Read the model definition and answer for the solid it produces. Units are mm, in the model's axes. Face numbers are marked on the shaded views. A direction names the side the tool comes from. Give positions to 0.01 mm unless a question says otherwise; leave off trailing zeros. Loops run counter-clockwise (first coordinate to the right, second up) from the corner with the lowest first, then second, coordinate; pieces in that order, holes last. Notation, with made-up numbers: (-29.5, 54.5) - (-1.5, 54.5) arc R21 ccw to (-1.5, 90.5) - close; hole circle Ø5 at (50.5, 5). An arc over 180 degrees is marked (long way). Use a Markdown table: item, result. Add a question column.
Item 1: Each of these flat-tipped pins is pushed along its axis until it touches: P1, Ø1.9, axis at x = -4.5, y = 4, coming from the +Z side; P2, Ø8, axis at x = -2, y = 3, coming from the +Z side; P3, Ø12, axis at x = 6, z = 18.5, coming from the +Y side. Where does it stop, or does it pass through?
Item 2: A cutting plane is placed at C-C (y = -14). Determine the outline of the cut face in (x, z), plus the area to 3 significant figures.
Item 3: Which of the six approach directions +Z, -Z, +X, -X, +Y, -Y give full straight-line access (tool end or side, diameter ignored) to the marked faces 4 and 5?
Item 4: A cutting plane is placed at A-A (z = 7). Determine the outline of the cut face in (x, y).
Item 5: A cutting plane is placed at B-B (z = 22). Determine the outline of the cut face in (x, y).
Item 6: A cutting plane is placed at D-D (x = -5). Determine the outline of the cut face in (y, z), plus the area to 3 significant figures.
Item 7: Consider probe 1 along Y at (x, z) = (0, 5.25); probe 2 along X at (y, z) = (-27.65, 14); probe 3 along X at (y, z) = (-18, 13). Determine where each line is inside the solid, lowest interval first. Write a range as [from, to].
Item 8: For a pull along X with two mould halves and no side action, classify the marked faces 1, 2 and 3 as +X half, -X half, draft (parallel to the pull), parting line (faces both ways), or undercut.
from build123d import *

# Parameters (mm, degrees)
SKETCH1_R           = 6.5
BOSS_EXTRUDE1_DEPTH = 13
CUT_EXTRUDE1_DEPTH  = 2
SKETCH3_R           = 1
SKETCH3_W           = 13
SKETCH3_H           = 22
CUT_EXTRUDE2_DEPTH  = 9
BOSS_EXTRUDE2_DEPTH = 18
BOSS_EXTRUDE3_DEPTH = 1.5
BOSS_EXTRUDE4_DEPTH = 1.5
SKETCH7_R           = 2.5
SKETCH7_R_2         = 1.3
CUT_EXTRUDE3_DEPTH  = 5


with BuildPart() as part:
    # Sketch1 → Boss-Extrude1 (new body)
    with BuildSketch(Plane.XY):
        with BuildLine():
            Line((-16.5, 0), (-16.5, -29.5))
            Line((-16.5, -29.5), (16.5, -29.5))
            Line((16.5, -29.5), (16.5, 0))
            ThreePointArc((16.5, 0), (0, 16.5), (-16.5, 0))
        make_face()
        with Locations(Location((0, 0, 0), (0, 0, 180))):
            Circle(SKETCH1_R, mode=Mode.SUBTRACT)
    extrude(amount=BOSS_EXTRUDE1_DEPTH)

    # Sketch2 → Cut-Extrude1 (cut)
    with BuildSketch(Plane.XY.offset(13)):
        with BuildLine():
            Line((-13.5, -26.5), (13.5, -26.5))
            Line((13.5, -26.5), (13.5, 0))
            ThreePointArc((13.5, 0), (0, 13.5), (-13.5, 0))
            Line((-13.5, 0), (-13.5, -26.5))
        make_face()
    extrude(amount=-CUT_EXTRUDE1_DEPTH, mode=Mode.SUBTRACT)

    # Sketch3 → Cut-Extrude2 (cut)
    with BuildSketch(Plane.XY.offset(11)):
        with Locations((0, 9.3)):
            Circle(SKETCH3_R)
        with Locations(Location((0, -18.3, 0), (0, 0, 180))):
            Circle(SKETCH3_R)
        with Locations((0, -4.5)):
            Rectangle(SKETCH3_W, SKETCH3_H)
    extrude(amount=-CUT_EXTRUDE2_DEPTH, mode=Mode.SUBTRACT)

    # Sketch4 → Boss-Extrude2 (add)
    with BuildSketch(Plane.XY.offset(13)):
        Polygon((-16.5, -26.5), (-16.5, -29.5), (16.5, -29.5), (16.5, -26.5), (13.5, -26.5), (-13.5, -26.5), align=None)
    extrude(amount=BOSS_EXTRUDE2_DEPTH)

    # Sketch5 → Boss-Extrude3 (add, symmetric)
    with BuildSketch(Plane(origin=(-15, 0, 0), x_dir=(0, 0, -1), z_dir=(1, 0, 0))):
        Polygon((-13, 0), (-31, -26.5), (-13, -26.5), align=None)
    extrude(amount=BOSS_EXTRUDE3_DEPTH, both=True)

    # Sketch6 → Boss-Extrude4 (add, symmetric)
    with BuildSketch(Plane(origin=(15, 0, 0), x_dir=(0, 0, -1), z_dir=(1, 0, 0))):
        Polygon((-13, 0), (-31, -26.5), (-13, -26.5), align=None)
    extrude(amount=BOSS_EXTRUDE4_DEPTH, both=True)

    # Sketch7 → Cut-Extrude3 (cut)
    with BuildSketch(Plane.XZ.offset(29.5)):
        with Locations(Location((-5, 14, 0), (0, 0, 270))):
            Circle(SKETCH7_R)
        with Locations(Location((-0.5, 14, 0), (0, 0, 270))):
            Circle(SKETCH7_R_2)
        with Locations(Location((-9.5, 14, 0), (0, 0, 270))):
            Circle(SKETCH7_R_2)
    extrude(amount=-CUT_EXTRUDE3_DEPTH, mode=Mode.SUBTRACT)


solid = part.part
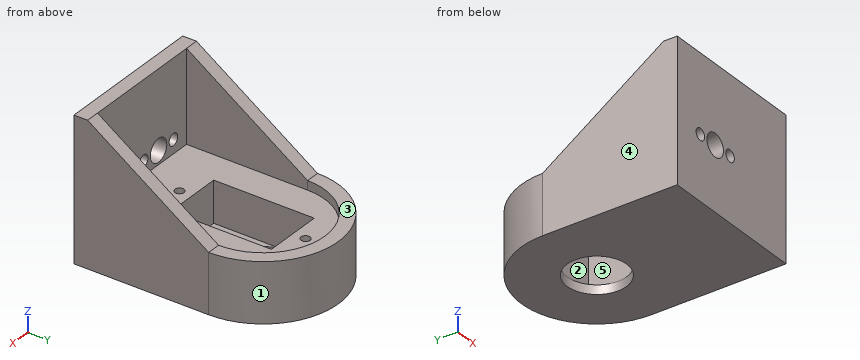
Geometry says:
| question | item | result |
|---|---|---|
| 1 | P1 | z = 2 |
| 1 | P2 | z = 11 |
| 1 | P3 | y = 16.1 |
| 2 | outline | (-16.5, 0) - (16.5, 0) - (16.5, 22.51) - (13.5, 22.51) - (13.5, 11) - (6.5, 11) - (6.5, 2) - (-6.5, 2) - (-6.5, 11) - (-13.5, 11) - (-13.5, 22.51) - (-16.5, 22.51) - close |
| 2 | area | 315 mm² |
| 3 | face 4 | +Z, -Z, -X, +Y, -Y |
| 3 | face 5 | +Z |
| 4 | outline | (-16.5, -29.5) - (16.5, -29.5) - (16.5, 0) arc R16.5 ccw to (-16.5, 0) - close; hole (-6.5, -15.5) - (6.5, -15.5) - (6.5, 6.5) - (-6.5, 6.5) - close; hole circle Ø2 at (0, -18.3); hole circle Ø2 at (0, 9.3) |
| 5 | outline | (-16.5, -29.5) - (16.5, -29.5) - (16.5, -13.25) - (13.5, -13.25) - (13.5, -26.5) - (-13.5, -26.5) - (-13.5, -13.25) - (-16.5, -13.25) - close |
| 6 | outline | (-29.5, 0) - (-4.15, 0) - (-4.15, 2) - (-15.5, 2) - (-15.5, 11) - (-26.5, 11) - (-26.5, 11.5) - (-29.5, 11.5) - close; (-29.5, 16.5) - (-26.5, 16.5) - (-26.5, 31) - (-29.5, 31) - close; (4.15, 0) - (15.72, 0) - (15.72, 13) - (12.54, 13) - (12.54, 11) - (6.5, 11) - (6.5, 2) - (4.15, 2) - close |
| 6 | area | 334 mm² |
| 7 | probe 1 | [-29.5, -19.3], [-17.3, -15.5], [6.5, 8.3], [10.3, 16.5] |
| 7 | probe 2 | [-16.5, -10.8], [-8.2, -7.5], [-2.5, -1.8], [0.8, 16.5] |
| 7 | probe 3 | [-16.5, -13.5], [13.5, 16.5] |
| 8 | face 1 | parting line |
| 8 | face 2 | undercut |
| 8 | face 3 | draft |
